Work out the finished part from the listing and answer in its coordinate system (mm). A direction names the side the tool comes from. Give positions to 0.01 mm unless a question says otherwise; leave off trailing zeros. Order: outer loops, then holes, each group sorted by start corner. A loop starts at its lowest first (then second) coordinate and runs counter-clockwise, first axis right, second up. Notation, with made-up numbers: M 14,10.25 L 31,10.25 A17 ccw 31,39.25 Z; hole C 60.5,63.25 d1. An arc over 180 degrees is marked long. One line per item, written item: value.
from build123d import *

# Parameters (mm, degrees)
F0_W     = 17.197048
F0_H     = 11
F1_DEPTH = 25.4


with BuildPart() as f1:
    # F0 (on Front) → F1 (new body)
    with BuildSketch(Plane.XZ):
        Polygon((-40.64, -5.5), (40.64, -5.5), (40.64, 5.5), (26.59588, 5.5), (9.398832, 5.5), (-7.796968, 5.5), (-24.994018, 5.5), (-40.64, 5.5), align=None)
        Polygon((-40.64, 49.5), (-40.64, 5.5), (-24.994018, 5.5), (-24.994018, 38.5), (-24.994018, 49.5), align=None)
        with Locations((17.997356, 11)):
            Rectangle(F0_W, F0_H)
        Polygon((-24.994018, 38.5), (-24.994018, 5.5), (-7.796968, 5.5), (-7.796968, 27.5), (-7.796968, 38.5), align=None)
        Polygon((-7.796968, 5.5), (9.398832, 5.5), (9.398832, 16.5), (9.398832, 27.5), (-7.796968, 27.5), align=None)
    extrude(amount=F1_DEPTH)


solid = f1.part
(1) Given P1, Ø1, axis at y = -5, z = 6.5, coming from the +X side; P2, Ø3, axis at y = -4, z = 30.5, coming from the +X side; P3, Ø2, axis at x = 29, y = -7.5, coming from the +Z side, each flat-ended and moving along its own axis, determine where each tip first touches the part or whether it passes through.
Findings:
P1: stops at x = 26.6
P2: stops at x = -7.8
P3: stops at z = 5.5
(2) Find the intervals of material crossed by probe 1 along Z at (x, y) = (-15, -14); probe 2 along X at (y, z) = (-6.5, 21.5); probe 3 along Z at (x, y) = (36, -9.25), in increasing order. Write a range as from..to.
Findings:
probe 1: z = -5.5..38.5
probe 2: x = -40.64..9.4
probe 3: z = -5.5..5.5
(3) Section A-A, the plane y = -16 is taken. Give the vertices of the cut face in (x, z).
Findings:
outline: M -40.64,-5.5 L 40.64,-5.5 L 40.64,5.5 L 26.6,5.5 L 26.6,16.5 L 9.4,16.5 L 9.4,27.5 L -7.8,27.5 L -7.8,38.5 L -24.99,38.5 L -24.99,49.5 L -40.64,49.5 Z
(4) Section B-B, the plane z = 26 is taken. Give the vertices of the cut face in (x, y).
Findings:
outline: M -40.64,-25.4 L 9.4,-25.4 L 9.4,0 L -40.64,0 Z
(5) Which of the six approach directions +Z, -Z, +X, -X, +Y, -Y give full straight-line access (tool end or side, diameter ignored) to faces 1 (the flat face through (-24.994, -13, 44)), 2 (the flat face through (-10, -25.4, 16))?
Findings:
face 1: +Z, +X, +Y, -Y
face 2: +Z, -Z, +X, -X, -Y
(6) Section C-C, the plane x = -23 is taken. Give the vertices of the cut face in (y, z), then the cut area to 3 significant figures.
Findings:
outline: M -25.4,-5.5 L 0,-5.5 L 0,38.5 L -25.4,38.5 Z
area: 1,120 mm^2
